Check sheet for the drawn part. Datum: minimum x, y, z corner. Units: mm. Give positions to 0.01 mm unless a question says otherwise; leave off trailing zeros. Order: outer loops, then holes, each group sorted by start corner. A loop starts at its lowest first (then second) coordinate and runs counter-clockwise, first axis right, second up. Notation, with made-up numbers: (7.25, 38) -> (56.25, 38) arc R24 ccw to (56.25, 52) -> close; hole circle Ø9 at (83, 76.25). An arc over 180 degrees is marked (long way). Return JSON: item names as keys, results as strings. Group by question number.
(1) Thickness scan on line 1 along Z through (x, y) = (165, 4); line 2 along X through (y, z) = (1.75, 5); line 3 along Y through (x, z) = (116.5, 79). Record the ranges inside material, lowest first.
(2) Cross-section at A-A on z = 115. Enter the section's corners in (x, y), then the cut area to 3 significant figures.
(3) Depth check by flat-ended pin: pin 1 Ø8 at (y, z) = (8.5, 37.5) entering from -X; pin 2 Ø2 at (y, z) = (9.5, 39.5) entering from -X; pin 3 Ø2 at (x, z) = (40, 39.5) entering from +Y; pin 4 Ø4 at (x, y) = (36, 14) entering from -Z (3 decimals). Enter the tip coordinate at first touch or a pass-through.
(4) Cross-section at C-C on x = 17.5. Enter the section's corners in (y, z) (1 decimal), then the cut area to 3 significant figures.
(5) Cross-section at B-B on x = 165. Enter the section's corners in (y, z).
(6) Cross-section at D-D on z = 33. Enter the section's corners in (x, y).
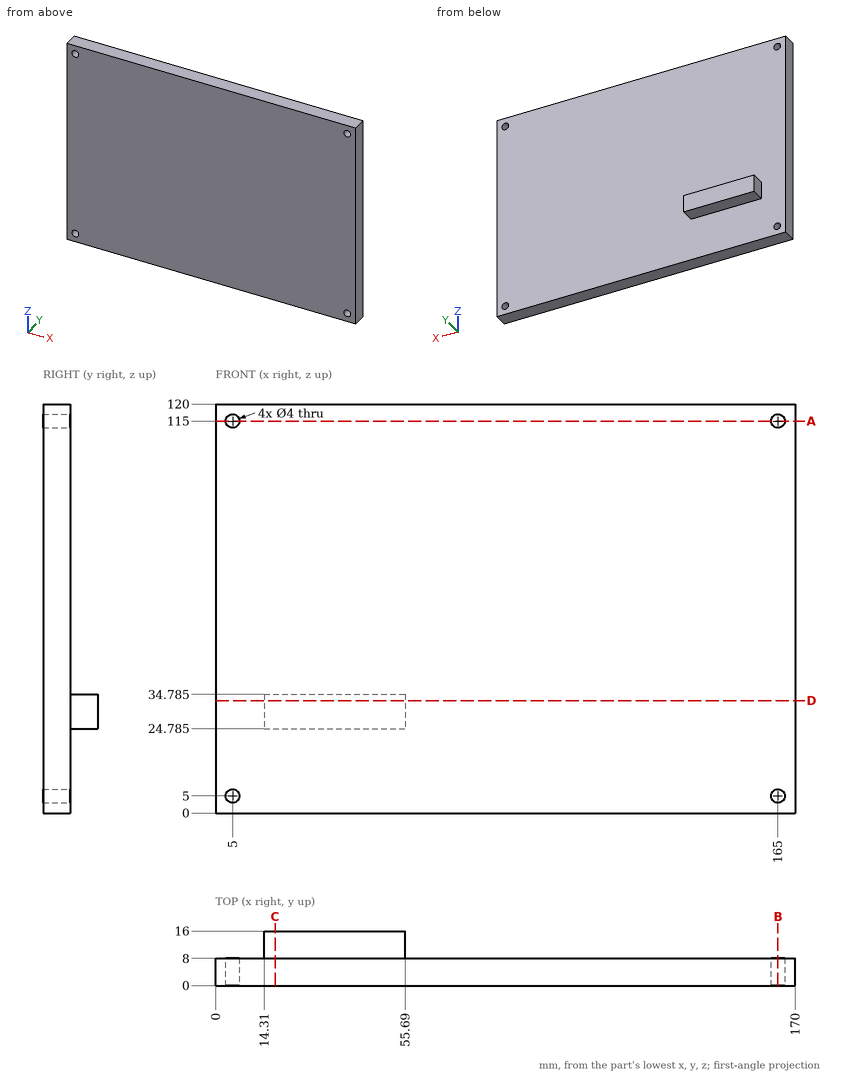
Verdict:
{
 "1": {"line 1": "0 to 3, 7 to 113, 117 to 120", "line 2": "0 to 3, 7 to 163, 167 to 170", "line 3": "0 to 8"},
 "2": {"outline": "(0, 0) -> (3, 0) -> (3, 8) -> (0, 8) -> close; (7, 0) -> (163, 0) -> (163, 8) -> (7, 8) -> close; (167, 0) -> (170, 0) -> (170, 8) -> (167, 8) -> close", "area": "1,300 mm²"},
 "3": {"pin 1": "x = 0", "pin 2": "through", "pin 3": "y = 8", "pin 4": "z = 24.785"},
 "4": {"outline": "(0, 0) -> (8, 0) -> (8, 24.8) -> (16, 24.8) -> (16, 34.8) -> (8, 34.8) -> (8, 120) -> (0, 120) -> close", "area": "1,040 mm²"},
 "5": {"outline": "(0, 0) -> (8, 0) -> (8, 3) -> (0, 3) -> close; (0, 7) -> (8, 7) -> (8, 113) -> (0, 113) -> close; (0, 117) -> (8, 117) -> (8, 120) -> (0, 120) -> close"},
 "6": {"outline": "(0, 0) -> (170, 0) -> (170, 8) -> (55.69, 8) -> (55.69, 16) -> (14.31, 16) -> (14.31, 8) -> (0, 8) -> close"}
}
